Check sheet for the drawn part. Datum: minimum x, y, z corner. Units: mm. A direction names the side the tool comes from. Coordinates: 2 decimals unless noted, no trailing zeros. Loops run counter-clockwise (first coordinate to the right, second up) from the corner with the lowest first, then second, coordinate; pieces in that order, holes last.
Q1. Go/stop test with flat-tipped pins: P1, Ø2, axis at x = 342.5, y = 997, coming from the -Z side; P2, Ø7.5, axis at x = 588, y = 26, coming from the -Z side; P3, Ø8, axis at x = 559, z = 594, coming from the +Y side. Record where each tip stops, or that it passes through.
Q2. Access from +Z, -Z, +X, -X, +Y, -Y to the whole of each face (thin tool, end or side, straight path). Record for the marked faces 1 and 2.
Q3. Sectioned sample at A-A (x = 514). Enter the section's corners in (y, z), then the cut area to 3 significant figures.
Q4. Sectioned sample at B-B (z = 63). Enter the section's corners in (x, y).
Q5. Material ranges on probe 1 along Y at (x, z) = (248.5, 594); probe 2 along Z at (x, y) = (410, 793.5), recorded low to high.
Q6. Sectioned sample at C-C (y = 1058). Enter the section's corners in (x, z).
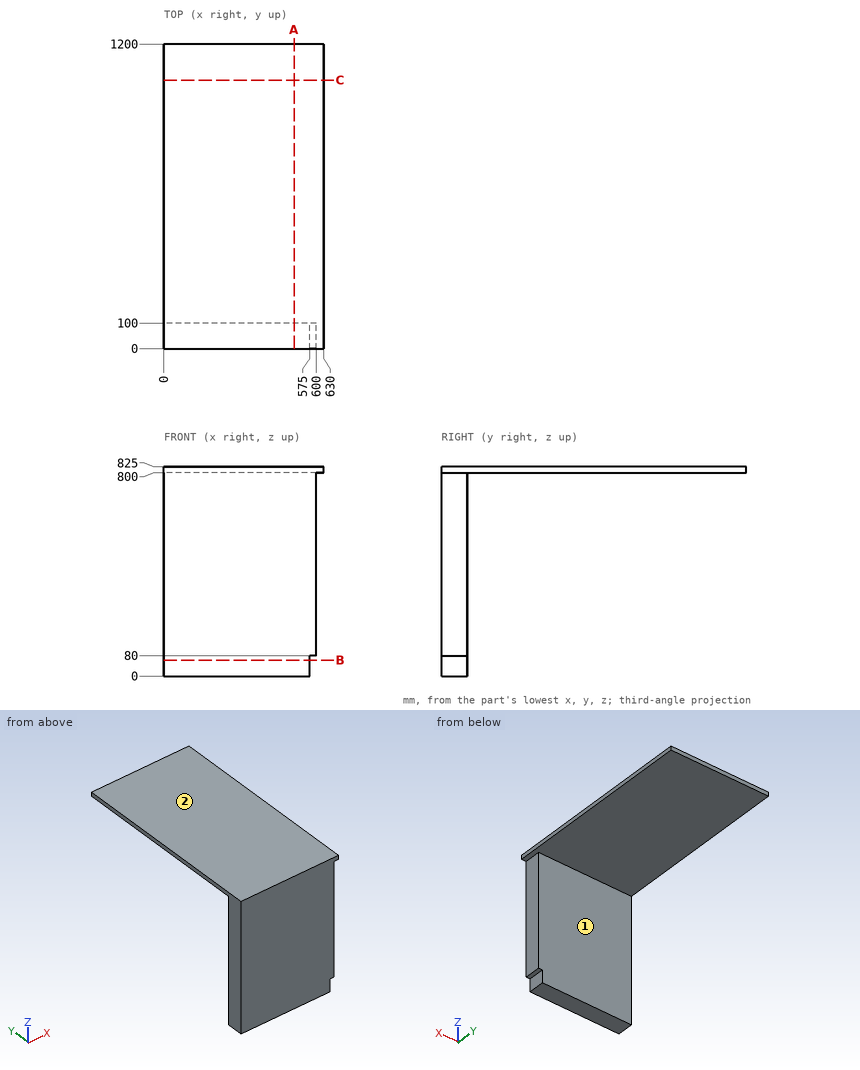
Geometry check:
1. P1: stops at z = 800
1. P2: stops at z = 80
1. P3: stops at y = 100
2. face 1: -Z, +X, -X, +Y
2. face 2: +Z, +X, -X, +Y, -Y
3. outline: (0, 0) - (100, 0) - (100, 800) - (1200, 800) - (1200, 825) - (0, 825) - close
3. area: 110,000 mm2
4. outline: (0, 0) - (575, 0) - (575, 100) - (0, 100) - close
5. probe 1: y = 0 to 100
5. probe 2: z = 800 to 825
6. outline: (0, 800) - (630, 800) - (630, 825) - (0, 825) - close
